Source: CAD feature listing. Evaluate the final solid. Frame: model axes, mm. Face numbers are marked on the shaded views. A direction names the side the tool comes from. Coordinates: 2 decimals unless noted, no trailing zeros. Order: outer loops, then holes, each group sorted by start corner. A loop starts at its lowest first (then second) coordinate and runs counter-clockwise, first axis right, second up. Notation, with made-up numbers: (-22, 23.5) - (24, 23.5) arc R21 ccw to (24, 60.5) - close; hole circle Ø5 at (65.5, 23). An arc over 180 degrees is marked (long way). One line per question, with ' | ' between items.
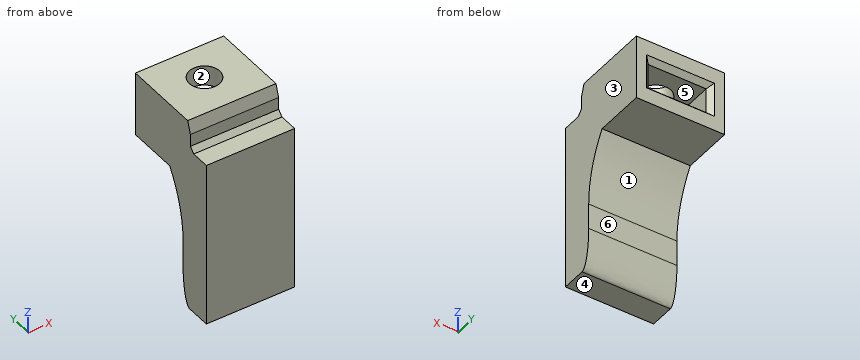
from build123d import *

# Parameters (mm, degrees)
RESSALTO_EXTRUS_O1_DEPTH = 9
CHANFRO5_SIZE            = 1
CHAMFER1_SIZE            = 0.8
CHAMFER1_SIZE2           = 2.46214683
ESBO_O3_R                = 3.1
CORTE_EXTRUS_O1_DEPTH    = 10.7
CORTE_EXTRUS_O4_START    = -4
CORTE_EXTRUS_O4_DEPTH    = 5.1
CHAMFER2_SIZE            = 1
FILETE1_SIZE             = 2
FILETE1_SIZE_2           = 8


with BuildPart() as part:
    # Esboço2 → Ressalto-extrusão1 (new, symmetric)
    with BuildSketch(Plane(origin=(0, 0, 0), x_dir=(0, 0, -1), z_dir=(1, 0, 0))):
        with BuildLine():
            Line((0, 0), (0, -16.5))
            Line((0, -16.5), (6, -16.5))
            Line((6, -16.5), (6, -21.3))
            Line((6, -21.3), (40, -21.3))
            Line((40, -21.3), (40, -14.3))
            Line((40, -14.3), (26.764659966, -14.3))
            ThreePointArc((26.764659966, -14.3), (19.693592154, -13.279157617), (13.2, -10.3))
            Line((13.2, -10.3), (13.2, 0))
            Line((13.2, 0), (0, 0))
        make_face()
    extrude(amount=RESSALTO_EXTRUS_O1_DEPTH, both=True)

    # Chanfro5
    chanfro5_edges = [part.edges().sort_by_distance(p)[0] for p in [
        (0, -16.5, -6),
    ]]
    chamfer(chanfro5_edges, length=CHANFRO5_SIZE)

    # Chamfer1
    chamfer1_edges = [part.edges().sort_by_distance(p)[0] for p in [
        (0, -16.5, 0),
    ]]
    chamfer1_side = [part.faces().sort_by_distance(p)[0] for p in [
        (0, -8.25, 0),
    ]]
    chamfer(chamfer1_edges, length=CHAMFER1_SIZE, length2=CHAMFER1_SIZE2, reference=chamfer1_side[0])

    # Esboço3 → Corte-extrusão1 (cut)
    with BuildSketch(Plane(origin=(0, 0, 0), x_dir=(-1, 0, 0), z_dir=(0, 0, -1))):
        with Locations(Location((0, -7.5, 0), (0, 0, 180))):
            Circle(ESBO_O3_R)
    extrude(amount=CORTE_EXTRUS_O1_DEPTH, mode=Mode.SUBTRACT)

    # Esboço7 → Corte-extrusão4 (cut)
    with BuildSketch(Plane(origin=(0, 0, -13.2), x_dir=(-1, 0, 0), z_dir=(0, 0, -1)).offset(CORTE_EXTRUS_O4_START)):
        Polygon((2.95892013, -2.375), (5.917840259, -7.5), (5.917840259, 0), (-5.917840259, 0), (-5.917840259, -7.5), (-2.95892013, -2.375), align=None)
        Polygon((2.95892013, -12.625), (5.917840259, -7.5), (2.95892013, -2.375), (-2.95892013, -2.375), (-5.917840259, -7.5), (-2.95892013, -12.625), align=None)
    extrude(amount=-CORTE_EXTRUS_O4_DEPTH, mode=Mode.SUBTRACT)

    # Chamfer2
    chamfer2_edges = [part.edges().sort_by_distance(p)[0] for p in [
        (0, 0, -4.1),
        (5.917840259, 0, -6.65),
        (-5.917840259, 0, -6.65),
        (0, 0, -9.2),
    ]]
    chamfer(chamfer2_edges, length=CHAMFER2_SIZE)

    # Filete1
    # an asymmetric fillet: 8, 2 mm, written as the material it takes off along each edge
    with BuildSketch(Plane(origin=(-29, -14.3, -40), x_dir=(0, -1, 0), z_dir=(1, 0, 0))) as filete1_piece_1:
        with BuildLine():
            Bezier((FILETE1_SIZE, 0), (0, 0), (0, -FILETE1_SIZE_2), weights=[1, 0.707106781, 1])
            Line((0, -FILETE1_SIZE_2), (0, 0))
            Line((0, 0), (FILETE1_SIZE, 0))
        make_face()
    extrude(amount=58, mode=Mode.SUBTRACT)


solid = part.part
(1) Cut plane D-D (y = -18.25). Return the cut outline in (x, z).
Taken from the geometry:
outline: (-9, -40) - (9, -40) - (9, -6) - (-9, -6) - close
(2) Pull-direction query (Y, two-part tool) for the marked faces 1, 2 and 3; classes: pulls with the +Y half, pulls with the -Y half, needs draft (parallel to the pull), parting line crosses it, or undercut.
Taken from the geometry:
face 1: pulls with the +Y half | face 2: undercut | face 3: needs draft
(3) Pin query (flat end, axial travel): P1, Ø2.5, axis at x = -1, z = -7.5, coming from the +Y side (3 decimals); P2, Ø10, axis at x = -6, y = -5, coming from the -Z side; P3, Ø10, axis at x = 0.5, y = -5.5, coming from the -Z side; P4, Ø10, axis at x = 3, y = -16, coming from the -Z side. Return the tip coordinate at first contact, or that it passes through.
Taken from the geometry:
P1: stops at y = -12.625 | P2: stops at z = -13.2 | P3: stops at z = -13.51 | P4: stops at z = -40
(4) Cut plane B-B (y = -6.75). Return the cut outline in (x, z).
Taken from the geometry:
outline: (-9, -13.2) - (9, -13.2) - (9, 0) - (3.01, 0) - (3.01, -4.1) - (5.92, -4.1) - (5.92, -9.2) - (3.01, -9.2) - (3.01, -10.7) - (-3.01, -10.7) - (-3.01, -9.2) - (-5.92, -9.2) - (-5.92, -4.1) - (-3.01, -4.1) - (-3.01, 0) - (-9, 0) - close
(5) Cut plane A-A (y = -1.75). Return the cut outline in (x, z).
Taken from the geometry:
outline: (-9, -13.2) - (9, -13.2) - (9, 0) - (-9, 0) - close; hole (-5.92, -9.2) - (5.92, -9.2) - (5.92, -4.1) - (-5.92, -4.1) - close
(6) Material intervals for L1, parallel to X at y = -7.5, z = -1.45; L2, parallel to Y at x = 0, z = -10.3; L3, parallel to Z at x = -3.5, y = -10.25, sorted ascending. Write a range as from..to.
Taken from the geometry:
L1: x = -9..-3.1, 3.1..9 | L2: y = -21.3..-10.6, -4.4..0 | L3: z = -13.2..-9.2, -4.1..0
(7) Cut plane C-C (z = -23). Return the cut outline in (x, y), and give its area (3 significant figures).
Taken from the geometry:
outline: (-9, -21.3) - (9, -21.3) - (9, -14.01) - (-9, -14.01) - close | area: 131 mm²
(8) Set-up query: the marked faces 4, 5 and 6. Return all of +Z, -Z, +X, -X, +Y, -Y with unobstructed straight access to the full face (end or side cutting, diameter ignored); none if empty.
Taken from the geometry:
face 4: -Z, +X, -X, +Y, -Y | face 5: +Y | face 6: -Z, +X, -X, +Y
